Could you check a few things on this drawing? It's one solid part, dimensions in mm from its lowest x, y, z. Round coordinates to 2 decimals unless told otherwise and drop trailing zeros. Write each loop counter-clockwise with the first axis right and the second up, starting at its lowest first coordinate (ties: lowest second). Pieces come first, ordered by that corner, then holes. Notation, with made-up numbers: (69.25, 26.5) -> (74.25, 26.5) arc R30 ccw to (74.25, 53.5) -> close; hole circle Ø7 at (72, -17). An arc over 180 degrees is marked (long way). Answer in a Markdown table with one row per item.
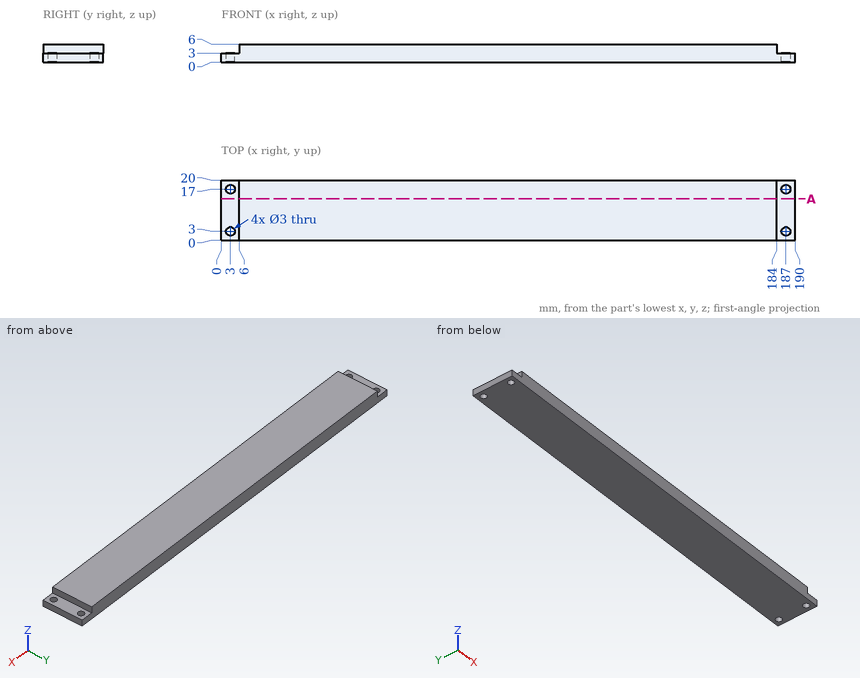
1) For pin 1 (6.5 mm diameter, centred on x = 188, y = 7, fed in from +Z); pin 2 (1.5 mm diameter, centred on y = 13.5, z = 4.5, fed in from +X); pin 3 (3.5 mm diameter, centred on y = 15, z = 5, fed in from -X), each with a flat end and sliding along its axis, tell me the tip position at first contact or that it passes through.
Response:
| item | result |
|---|---|
| pin 1 | stops at z = 3 |
| pin 2 | stops at x = 184 |
| pin 3 | stops at x = 6 |
2) I need wall thicknesses on line 1 (Y direction, x = 187, z = 2.2); line 2 (X direction, y = 3.25, z = 1.9); line 3 (X direction, y = 4.25, z = 2.35). Which ranges of each line are inside material? Lowest first, please. Write a range as [from, to].
Response:
| item | result |
|---|---|
| line 1 | y = [0, 1.5], [4.5, 15.5], [18.5, 20] |
| line 2 | x = [0, 1.52], [4.48, 185.52], [188.48, 190] |
| line 3 | x = [0, 2.17], [3.83, 186.17], [187.83, 190] |
3) I want a section at A-A, the plane y = 13.75. List the corners of the cut face in (x, z) for me, and give its area (3 significant figures).
Response:
| item | result |
|---|---|
| outline | (0, 0) -> (190, 0) -> (190, 3) -> (184, 3) -> (184, 6) -> (6, 6) -> (6, 3) -> (0, 3) -> close |
| area | 1,100 mm^2 |
